Part model, mm, in its own coordinate system. A direction names the side the tool comes from. Coordinates: 2 decimals unless noted, no trailing zeros. Loops run counter-clockwise (first coordinate to the right, second up) from the corner with the lowest first, then second, coordinate; pieces in that order, holes last. Notation, with made-up numbers: (56, -20) - (67, -20) arc R17 ccw to (67, -14) - close; hole circle Ø2 at (67.5, 36.25). An arc over 180 degrees is marked (long way). Use a Markdown table: item, result. Add a question column.
1) Tool access for faces 4 (the face through (1.5, -14, 22)), 5 (the face through (4, 0, 4)), 6 (the face through (13, -14, 18)), 7 (the face through (-10.4, -22.3, 2.5)), 8 (the face through (-14, -14, 5)): list every direction of +Z, -Z, +X, -X, +Y, -Y with a clear straight run to the whole face (end or side of a thin tool).
2) Drop flat-ended pins along their axis: P1, Ø1, axis at x = -3, z = 18, coming from the -Y side; P2, Ø6, axis at x = 13.5, y = -21.5, coming from the +Z side; P3, Ø6.5, axis at x = 12, y = -23.5, coming from the -Z side; P4, Ø3, axis at y = -11.5, z = 22, coming from the -X side. Give the stop position or say it passes through.
3) Band-saw the part on D-D (z = 9.25). Give the cut face in (x, y).
4) Band-saw the part on C-C (y = -17.75). Give the cut face in (x, z).
5) Band-saw the part on B-B (z = 3). Give the cut face in (x, y).
6) Probe probe 1 along Y at (x, z) = (12, 13); probe 2 along X at (y, z) = (-23.5, 3.4); probe 3 along X at (y, z) = (-4, 13.25). List the from-to ranges inside material, lowest first. Write a range as [from, to].
7) Band-saw the part on A-A (x = 12). Give the cut face in (y, z), plus the area to 3 significant figures.
8) Pull direction X, two halves, no side cores. Call faces 1 (the face through (4, -29, 4)), 2 (the face through (13.474, -6.852, 9.126)), 3 (the face through (-7.52, -14.3, 19.59)): +X half, -X half, draft (parallel to the pull), parting line (faces both ways), or undercut.
from build123d import *

# Parameters (mm, degrees)
F1_DEPTH = 29
F3_D     = 4


with BuildPart() as f1:
    # F0 (on Front) → F1 (new body)
    with BuildSketch(Plane.XZ):
        with BuildLine():
            Line((-17.5, 0), (0, 0))
            Line((0, 0), (17.5, 0))
            Line((17.5, 0), (17.5, 5))
            Line((17.5, 5), (10, 5))
            Line((10, 5), (10, 13))
            ThreePointArc((10, 13), (9.659258, 15.58819), (8.660254, 18))
            ThreePointArc((8.660254, 18), (5.637201, 21.259659), (1.5, 22.88686))
            Line((1.5, 22.88686), (1.5, 20.246378))
            ThreePointArc((1.5, 20.246378), (7.361494, 12.246077), (0, 5.6))
            ThreePointArc((0, 5.6), (-7.361494, 12.246077), (-1.5, 20.246378))
            Line((-1.5, 20.246378), (-1.5, 22.88686))
            ThreePointArc((-1.5, 22.88686), (-7.582875, 19.519202), (-10, 13))
            Line((-10, 13), (-10, 5))
            Line((-10, 5), (-17.5, 5))
            Line((-17.5, 5), (-17.5, 0))
        make_face()
        with BuildLine():
            Line((10, 5), (17.5, 5))
            Line((17.5, 5), (17.5, 18))
            Line((17.5, 18), (8.660254, 18))
            ThreePointArc((8.660254, 18), (9.659258, 15.58819), (10, 13))
            Line((10, 13), (10, 5))
        make_face()
    extrude(amount=F1_DEPTH)

    # F3 (through all)
    with Locations(Plane(origin=(0, 0, 0), x_dir=(1, 0, 0), z_dir=(0, 0, -1))):
        with Locations((-12, 23.5), (12, 23.5), (-12, 5.5), (12, 5.5)):
            Hole(F3_D / 2)


solid = f1.part
Answer block:
| question | item | result |
|---|---|---|
| 1 | face 4 | +Z, +Y, -Y |
| 1 | face 5 | +Z, -Z, +X, -X, +Y |
| 1 | face 6 | +Z, +X, +Y, -Y |
| 1 | face 7 | +Z, -Z |
| 1 | face 8 | +Z, -X, +Y, -Y |
| 2 | P1 | through |
| 2 | P2 | z = 18 |
| 2 | P3 | z = 0 |
| 2 | P4 | x = -6.61 |
| 3 | outline | (-10, -29) - (-6.38, -29) - (-6.38, 0) - (-10, 0) - close; (6.38, -29) - (17.5, -29) - (17.5, 0) - (6.38, 0) - close; hole circle Ø4 at (12, -23.5); hole circle Ø4 at (12, -5.5) |
| 4 | outline | (-17.5, 0) - (17.5, 0) - (17.5, 18) - (8.66, 18) arc R10 ccw to (1.5, 22.89) - (1.5, 20.25) arc R7.4 cw (long way) to (-1.5, 20.25) - (-1.5, 22.89) arc R10 ccw to (-10, 13) - (-10, 5) - (-17.5, 5) - close |
| 5 | outline | (-17.5, -29) - (17.5, -29) - (17.5, 0) - (-17.5, 0) - close; hole circle Ø4 at (-12, -23.5); hole circle Ø4 at (-12, -5.5); hole circle Ø4 at (12, -23.5); hole circle Ø4 at (12, -5.5) |
| 6 | probe 1 | [-29, -25.5], [-21.5, -7.5], [-3.5, 0] |
| 6 | probe 2 | [-17.5, -14], [-10, 10], [14, 17.5] |
| 6 | probe 3 | [-10, -7.4], [7.4, 10.68], [13.32, 17.5] |
| 7 | outline | (-29, 0) - (-25.5, 0) - (-25.5, 18) - (-29, 18) - close; (-21.5, 0) - (-7.5, 0) - (-7.5, 18) - (-21.5, 18) - close; (-3.5, 0) - (0, 0) - (0, 18) - (-3.5, 18) - close |
| 7 | area | 378 mm2 |
| 8 | face 1 | draft |
| 8 | face 2 | undercut |
| 8 | face 3 | -X half |
